```python
from build123d import *

# Parameters (mm, degrees)
SKETCH1_R           = 11.95
SKETCH1_R_2         = 1.25
BOSS_EXTRUDE5_DEPTH = 1
SKETCH1_9_R         = 1.25
BOSS_EXTRUDE9_DEPTH = 1
SKETCH1_12_R        = 1.025
CUT_EXTRUDE6_DEPTH  = 28.53713591


with BuildPart() as part:
    # Sketch1 → Boss-Extrude5 (new body)
    with BuildSketch(Plane.XY):
        Circle(SKETCH1_R)
        Circle(SKETCH1_R_2, mode=Mode.SUBTRACT)
    extrude(amount=BOSS_EXTRUDE5_DEPTH)

    # Sketch1_9 → Boss-Extrude9 (add)
    with BuildSketch(Plane.XY):
        Circle(SKETCH1_9_R)
    extrude(amount=BOSS_EXTRUDE9_DEPTH)

    # Sketch16 for Loft3 → Loft3 section 0
    with BuildSketch(Plane.XY.offset(1)):
        with BuildLine():
            Line((12.566853953, 12.883098649), (13.802379149, 12.169767844))
            add(Edge.make_bspline(
                [(1.079738119, 0.629813936), (10.901614273, 3.888080069), (13.802379149, 12.169767844)],
                knots=[0, 0, 0, 1, 1, 1], degree=2))
            # circular arc as an exact rational Bezier (weights 1, cos(half-angle), 1)
            Bezier((1.079738119, 0.629813936), (1.192655997, 0.436230196), (1.231288084, 0.215475415), weights=[1, 0.984305335, 1])
            add(Edge.make_bspline(
                [(1.231288084, 0.215475415), (8.568925474, -6.096520826), (17.440517686, -4.441665445)],
                knots=[0, 0, 0, 1, 1, 1], degree=2))
            Line((17.440517686, -4.441665445), (17.440517686, -5.868327054))
            add(Edge.make_bspline(
                [(1.085303928, -0.620173673), (8.817983248, -7.497034868), (17.440517686, -5.868327054)],
                knots=[0, 0, 0, 1, 1, 1], degree=2))
            Bezier((1.085303928, -0.620173673), (0.97411443, -0.814755294), (0.802251225, -0.958589053), weights=[1, 0.984305335, 1])
            add(Edge.make_bspline(
                [(0.802251225, -0.958589053), (-0.995279173, -10.469167557), (4.873663733, -17.324764093)],
                knots=[0, 0, 0, 1, 1, 1], degree=2))
            Line((4.873663733, -17.324764093), (3.638138537, -18.038094898))
            add(Edge.make_bspline(
                [(0.005565808, -1.249987609), (-2.083631025, -11.385114937), (3.638138537, -18.038094898)],
                knots=[0, 0, 0, 1, 1, 1], degree=2))
            Bezier((0.005565808, -1.249987609), (-0.218541567, -1.250985489), (-0.429036859, -1.174064467), weights=[1, 0.984305335, 1])
            add(Edge.make_bspline(
                [(-0.429036859, -1.174064467), (-9.564204647, -4.37264673), (-12.566853953, -12.883098649)],
                knots=[0, 0, 0, 1, 1, 1], degree=2))
            Line((-12.566853953, -12.883098649), (-13.802379149, -12.169767844))
            add(Edge.make_bspline(
                [(-1.079738119, -0.629813936), (-10.901614273, -3.888080069), (-13.802379149, -12.169767844)],
                knots=[0, 0, 0, 1, 1, 1], degree=2))
            Bezier((-1.079738119, -0.629813936), (-1.192655997, -0.436230196), (-1.231288084, -0.215475415), weights=[1, 0.984305335, 1])
            add(Edge.make_bspline(
                [(-1.231288084, -0.215475415), (-8.568925474, 6.096520826), (-17.440517686, 4.441665445)],
                knots=[0, 0, 0, 1, 1, 1], degree=2))
            Line((-17.440517686, 4.441665445), (-17.440517686, 5.868327054))
            add(Edge.make_bspline(
                [(-1.085303928, 0.620173673), (-8.817983248, 7.497034868), (-17.440517686, 5.868327054)],
                knots=[0, 0, 0, 1, 1, 1], degree=2))
            Bezier((-1.085303928, 0.620173673), (-0.97411443, 0.814755294), (-0.802251225, 0.958589053), weights=[1, 0.984305335, 1])
            add(Edge.make_bspline(
                [(-0.802251225, 0.958589053), (0.995279173, 10.469167557), (-4.873663733, 17.324764093)],
                knots=[0, 0, 0, 1, 1, 1], degree=2))
            Line((-4.873663733, 17.324764093), (-3.638138537, 18.038094898))
            add(Edge.make_bspline(
                [(-0.005565808, 1.249987609), (2.083631025, 11.385114937), (-3.638138537, 18.038094898)],
                knots=[0, 0, 0, 1, 1, 1], degree=2))
            Bezier((-0.005565808, 1.249987609), (0.218541567, 1.250985489), (0.429036859, 1.174064467), weights=[1, 0.984305335, 1])
            add(Edge.make_bspline(
                [(0.429036859, 1.174064467), (9.564204647, 4.37264673), (12.566853953, 12.883098649)],
                knots=[0, 0, 0, 1, 1, 1], degree=2))
        make_face()
    # Sketch22 for Loft3 → Loft3 section 1
    with BuildSketch(Plane.XY.offset(11)):
        with BuildLine():
            Line((13.128169943, 12.255599921), (14.324669046, 11.478584319))
            add(Edge.make_bspline(
                [(1.01550943, 0.620297101), (10.994449518, 3.360060613), (14.324669046, 11.478584319)],
                knots=[0, 0, 0, 1, 1, 1], degree=2))
            Bezier((1.01550943, 0.620297101), (1.118141168, 0.421068995), (1.145166898, 0.198594904), weights=[1, 0.984305335, 1])
            add(Edge.make_bspline(
                [(1.145166898, 0.198594904), (8.142403952, -6.488773235), (17.088446394, -5.300489037)],
                knots=[0, 0, 0, 1, 1, 1], degree=2))
            Line((17.088446394, -5.300489037), (17.013780694, -6.725195456))
            add(Edge.make_bspline(
                [(0.955648314, -0.628268735), (8.31782316, -7.900402598), (17.013780694, -6.725195456)],
                knots=[0, 0, 0, 1, 1, 1], degree=2))
            Bezier((0.955648314, -0.628268735), (0.834427583, -0.81676448), (0.655272233, -0.951406495), weights=[1, 0.984305335, 1])
            add(Edge.make_bspline(
                [(0.655272233, -0.951406495), (-1.637539933, -10.354875609), (3.86456559, -17.508233528)],
                knots=[0, 0, 0, 1, 1, 1], degree=2))
            Line((3.86456559, -17.508233528), (2.593400789, -18.155924345))
            add(Edge.make_bspline(
                [(-0.155571976, -1.200710406), (-2.772337218, -11.21260778), (2.593400789, -18.155924345)],
                knots=[0, 0, 0, 1, 1, 1], degree=2))
            Bezier((-0.155571976, -1.200710406), (-0.379424445, -1.189978045), (-0.585605526, -1.102145969), weights=[1, 0.984305335, 1])
            add(Edge.make_bspline(
                [(-0.585605526, -1.102145969), (-9.875654745, -3.818246944), (-13.319591664, -12.159889061)],
                knots=[0, 0, 0, 1, 1, 1], degree=2))
            Line((-13.319591664, -12.159889061), (-14.516090766, -11.382873459))
            add(Edge.make_bspline(
                [(-1.20693115, -0.524586241), (-11.185871238, -3.264349753), (-14.516090766, -11.382873459)],
                knots=[0, 0, 0, 1, 1, 1], degree=2))
            Bezier((-1.20693115, -0.524586241), (-1.309562888, -0.325358135), (-1.336588618, -0.102884044), weights=[1, 0.984305335, 1])
            add(Edge.make_bspline(
                [(-1.336588618, -0.102884044), (-8.333825672, 6.584484095), (-17.279868114, 5.396199897)],
                knots=[0, 0, 0, 1, 1, 1], degree=2))
            Line((-17.279868114, 5.396199897), (-17.205202415, 6.820906316))
            add(Edge.make_bspline(
                [(-1.147070034, 0.723979595), (-8.50924488, 7.996113458), (-17.205202415, 6.820906316)],
                knots=[0, 0, 0, 1, 1, 1], degree=2))
            Bezier((-1.147070034, 0.723979595), (-1.025849303, 0.91247534), (-0.846693953, 1.047117355), weights=[1, 0.984305335, 1])
            add(Edge.make_bspline(
                [(-0.846693953, 1.047117355), (1.446118213, 10.450586469), (-4.055987311, 17.603944388)],
                knots=[0, 0, 0, 1, 1, 1], degree=2))
            Line((-4.055987311, 17.603944388), (-2.784822509, 18.251635205))
            add(Edge.make_bspline(
                [(-0.035849744, 1.296421266), (2.580915498, 11.30831864), (-2.784822509, 18.251635205)],
                knots=[0, 0, 0, 1, 1, 1], degree=2))
            Bezier((-0.035849744, 1.296421266), (0.188002725, 1.285688905), (0.394183805, 1.197856829), weights=[1, 0.984305335, 1])
            add(Edge.make_bspline(
                [(0.394183805, 1.197856829), (9.684233025, 3.913957804), (13.128169943, 12.255599921)],
                knots=[0, 0, 0, 1, 1, 1], degree=2))
        make_face()
    loft()

    # Sketch1_12 → Cut-Extrude6 (cut, through all)
    with BuildSketch(Plane.XY):
        with Locations(Location((0, 0, 0), (0, 0, 180))):
            Circle(SKETCH1_12_R)
    extrude(amount=CUT_EXTRUDE6_DEPTH, mode=Mode.SUBTRACT)


solid = part.part
```
For this review, take the finished solid that the model builds, in its own axes (mm). A direction names the side the tool comes from. Give positions to 0.01 mm unless a question says otherwise; leave off trailing zeros.
1) Wall thickness on line 1 (Y direction, x = -3, z = 7.25); line 2 (Y direction, x = 2.5, z = 6.5); line 3 (X direction, y = -3, z = 10): over which ranges is each line inside the solid? List them lowest first.
2) For faces 4 (the face through (14, -5, 1)), 5 (the face through (12, 9, 1)), 6 (the face through (-12, -9, 1)), list the 3-axis set-ups (+Z, -Z, +X, -X, +Y, -Y) from which the entire face can be reached by the end or side of a thin tool; tool diameter is ignored.
3) Insertion check: pin 1 (3 mm diameter, centred on x = 13, z = 4.5, fed in from -Y); pin 2 (5 mm diameter, centred on x = -12.5, z = 9, fed in from -Y); pin 3 (2 mm diameter, centred on y = -13.5, z = 2.5, fed in from -X). Each pin has a flat end and moves straight along its axis. Give the tip position at first contact, or say it passes through.
4) The part is to be moulded in two halves that separate along Y. For faces 1 (the face through (6.42, 10.08, 0.49)), 2 (the face through (-14, 5, 1)), 3 (the face through (0.133, -1.016, 5.423)), say which applies: released by +Y, released by -Y, zero draft, split by the parting line, or undercut.
Derived:
1. line 1: y = -2.05 to -1.18, 1.29 to 2.32, 15.58 to 18.04
1. line 2: y = -17.37 to -14.77, -1.93 to -0.91, 1.1 to 1.95
1. line 3: x = -7.11 to -5.13, -0.54 to 0.27, 3.73 to 5.4
2. face 4: -Z, +X, -Y
2. face 5: -Z, +X, +Y
2. face 6: -Z, -X, -Y
3. pin 1: stops at y = -6.5
3. pin 2: stops at y = -12.48
3. pin 3: stops at x = -13.15
4. face 1: split by the parting line
4. face 2: zero draft
4. face 3: undercut
